```python
from build123d import *

# Parameters (mm, degrees)
F1_DEPTH = 24
F3_D     = 3.1
F6_D     = 8
F6_DEPTH = 26.9889453037
F7_R     = 3


with BuildPart() as f1:
    # F0 (on Front) → F1 (new body)
    with BuildSketch(Plane.XZ):
        with BuildLine():
            ThreePointArc((-14.5, 14.4879452037), (0, 28.9879452037), (14.5, 14.4879452037))
            Line((14.5, 14.4879452037), (14.5, 0))
            Line((14.5, 0), (25.5, 0))
            Line((25.5, 0), (18.4680759907, 20.7473516612))
            ThreePointArc((18.4680759907, 20.7473516612), (0, 33.9879452037), (-18.4680759907, 20.7473516612))
            Line((-18.4680759907, 20.7473516612), (-25.5, 0))
            Line((-25.5, 0), (-14.5, 0))
            Line((-14.5, 0), (-14.5, 14.4879452037))
        make_face()
    extrude(amount=F1_DEPTH)

    # F3 (through all)
    with Locations(Plane(origin=(0, 0, 0), x_dir=(1, 0, 0), z_dir=(0, 0, -1))):
        with Locations((-20, 12), (20, 12)):
            Hole(F3_D / 2)

    # F6 (through all, one way)
    with BuildSketch(Plane(origin=(0, 0, 7), x_dir=(1, 0, 0), z_dir=(0, 0, -1))):
        with Locations((-20, 12), (20, 12)):
            Circle(F6_D / 2)
    extrude(amount=-F6_DEPTH, mode=Mode.SUBTRACT)

    # F7
    f7_edges = [f1.edges().sort_by_distance(p)[0] for p in [
        (0, 0, 33.987945),
        (0, -24, 33.987945),
    ]]
    fillet(f7_edges, radius=F7_R)


solid = f1.part
```
Geometry: final body of the model. Coordinates: model frame, mm. A direction names the side the tool comes from. Round coordinates to 2 decimals unless told otherwise and drop trailing zeros. Order: outer loops, then holes, each group sorted by start corner. A loop starts at its lowest first (then second) coordinate and runs counter-clockwise, first axis right, second up. Notation, with made-up numbers: M -31.75,40.25 L 27.25,40.25 A17 ccw 27.25,53.25 Z; hole C -33,-31 d8. An arc over 180 degrees is marked long. Use one line per item in the form item = value. Start each with the question number.
Q1. Cut plane B-B (x = 0). Return loops of the section in (y, z), and give its area (3 significant figures).
Q2. Mould query, pull axis Y, two halves, no side actions, for faces 1 (the face through (18.568, -11.406, 3.549)), 2 (the face through (-14.5, -12, 7)), 3 (the face through (21.125, -0.902, 10.244)). Classes: +Y half, -Y half, draft (parallel to the pull), parting line (faces both ways), or undercut.
Q3. Cut plane A-A (y = -12). Return loops of the section in (x, z), and give its area (3 significant figures).
Q4. Cut plane C-C (y = -2). Return loops of the section in (x, z), and give its area (3 significant figures).
Q5. Pin query (flat end, axial travel): pin 1 Ø10.5 at (x, y) = (20, -12) entering from +Z; pin 2 Ø13 at (x, y) = (-20, -12) entering from +Z; pin 3 Ø5 at (x, y) = (7.5, -17) entering from -Z. Return the tip coordinate at first contact, or that it passes through.
Q6. Access query for faces 4 (the face through (20, -10, 7)), 5 (the face through (14.5, -12, 7)), 6 (the face through (15, -24, 13)). Directions: +Z, -Z, +X, -X, +Y, -Y. A direction counts if a zero-diameter tool reaches every point of the face in a straight line with its end or side. Return the directions, or none.
Q7. Material intervals for line 1 (X direction, y = -12, z = 4.5); line 2 (X direction, y = -12, z = 3.5); line 3 (Y direction, x = 20, z = 3.25), sorted ascending. Write a range as [from, to].
Geometry results:
q1.outline = M -24,28.99 L 0,28.99 L 0,30.99 A3 ccw -3,33.99 L -21,33.99 A3 ccw -24,30.99 Z
q1.area = 116 mm^2
q2.face_1 = undercut
q2.face_2 = draft
q2.face_3 = +Y half
q3.outline = M -25.5,0 L -21.55,0 L -21.55,7 L -23.13,7 Z; M -18.45,0 L -14.5,0 L -14.5,14.49 A14.5 cw 14.5,14.49 L 14.5,0 L 18.45,0 L 18.45,7 L 16,7 L 16,25.63 A19.5 ccw -16,25.63 L -16,7 L -18.45,7 Z; M 21.55,0 L 25.5,0 L 23.13,7 L 21.55,7 Z
q3.area = 330 mm^2
q4.outline = M -25.32,0 L -14.5,0 L -14.5,14.49 A14.5 cw 14.5,14.49 L 14.5,0 L 25.32,0 L 18.31,20.69 A19.33 ccw -18.31,20.69 Z
q4.area = 503 mm^2
q5.pin_1 = 27.24
q5.pin_2 = 28.56
q5.pin_3 = 24.99
q6.face_4 = +Z
q6.face_5 = -Z, +Y, -Y
q6.face_6 = +Z, -Z, +X, -X, -Y
q7.line_1 = [-23.97, -21.55], [-18.45, -14.5], [14.5, 18.45], [21.55, 23.97]
q7.line_2 = [-24.31, -21.55], [-18.45, -14.5], [14.5, 18.45], [21.55, 24.31]
q7.line_3 = [-24, -13.55], [-10.45, 0]
